Work out the finished part from the listing and answer in its coordinate system (mm). A direction names the side the tool comes from. Round coordinates to 2 decimals unless told otherwise and drop trailing zeros. Order: outer loops, then holes, each group sorted by start corner. A loop starts at its lowest first (then second) coordinate and runs counter-clockwise, first axis right, second up. Notation, with made-up numbers: (74.5, -26.75) -> (130.5, -26.75) arc R12 cw to (130.5, -20.75) -> close; hole circle Ø6 at (-38.75, 45.25). An arc over 180 degrees is marked (long way). Use one line per item in the form item = value.
```python
from build123d import *

# Parameters (mm, degrees)
F0_R     = 2
F2_W     = 4
F2_H     = 13
F3_DEPTH = 2
F5_DEPTH = 25


with BuildPart() as f1:
    # F0 (on Front) → F1 (revolve)
    with BuildSketch(Plane.XZ):
        with Locations((-18, 0)):
            Circle(F0_R)
    revolve(axis=Axis((0, 0, 11.250001), (0, 0, 1)))

    # F2 (on Top) → F3 (join, symmetric)
    with BuildSketch(Plane.XY):
        with Locations((2, -13.5)):
            Rectangle(F2_W, F2_H)
        with Locations((-2, -13.5)):
            Rectangle(F2_W, F2_H)
    extrude(amount=F3_DEPTH, both=True)

    # F4 (on face) → F5 (join)
    with BuildSketch(Plane.XZ.offset(20)):
        Polygon((0.5, 0.5), (2, 2), (0.5, 2), (0, 2), (-0.5, 2), (-2, 2), (-0.5, 0.5), (-0.5, -0.5), (-2, -2), (-0.5, -2), (0.5, -2), (2, -2), (0.5, -0.5), align=None)
        Polygon((2.070711, 1.929289), (2.141421, 2), (2, 2), (0.5, 0.5), (0.5, -0.5), (2, -2), (2.141421, -2), (2.070711, -1.929289), (0.6, -0.458579), (0.6, 0.458579), align=None)
        Polygon((-0.5, 0.5), (-2, 2), (-2.141421, 2), (-2.070711, 1.929289), (-0.6, 0.458579), (-0.6, -0.458579), (-2.070711, -1.929289), (-2.141421, -2), (-2, -2), (-0.5, -0.5), align=None)
    extrude(amount=F5_DEPTH)


solid = f1.part
```
Item 1: Consider line 1 along X through (y, z) = (-7.5, -1.1); line 2 along X through (y, z) = (-1, 1); line 3 along Y through (x, z) = (7, -0.6). Determine where each line is inside the solid, lowest interval first.
Findings:
line_1 = -18.18 to -14.51, -4 to 4, 14.51 to 18.18
line_2 = -19.71 to -16.24, 16.24 to 19.71
line_3 = -18.64 to -14.49, 14.49 to 18.64
Item 2: For faces 1 (the flat face through (0, -22, -2)), 2 (the flat face through (0, -7, 0)), 3 (the flat face through (-4, -19.8, 0.2)), 4 (the flat face through (0, -45, 0)), 5 (the flat face through (4, -19.8, 0.2)), determine the directions among +Z, -Z, +X, -X, +Y, -Y from which every point of the face is accessible in a straight line to the end or side of a thin tool.
Findings:
face_1 = -Z, +X, -X, +Y, -Y
face_2 = +Z, -Z
face_3 = -X, -Y
face_4 = +Z, -Z, +X, -X, -Y
face_5 = +X, -Y
Item 3: Flat-ended cylindrical pins translate along their axes: P1, Ø1.7, axis at x = -2, z = 0.5, coming from the -Y side; P2, Ø0.5, axis at y = -31.5, z = 0, coming from the -X side; P3, Ø1.2, axis at y = -10.5, z = 0, coming from the -X side. Find the tip coordinate at first contact, or state that the pin passes through.
Findings:
P1 = -20
P2 = -0.6
P3 = -17.38
Item 4: Determine the mould class of faces 6 (the flat face through (-4, -11, 0)), 7 (the flat face through (0, -22, 2)), 8 (the flat face through (3, -20, 0)) for opening direction Y: released by +Y, released by -Y, zero draft, split by the parting line, or undercut.
Findings:
face_6 = undercut
face_7 = zero draft
face_8 = released by -Y
Item 5: The part is cut by section A-A, the plane z = -1.25. Give the vertices of the cut face in (x, y), and give its area (3 significant figures).
Findings:
outline = (-4, -20) -> (-1.39, -20) -> (-1.39, -45) -> (1.39, -45) -> (1.39, -20) -> (4, -20) -> (4, -19.15) arc R19.56 ccw (long way) to (-4, -19.15) -> close; hole (-4, -15.94) -> (-4, -7) -> (4, -7) -> (4, -15.94) arc R16.44 ccw (long way) to start
area = 502 mm^2
Item 6: The part is cut by section B-B, the plane y = -8. Give the number of separate pieces and of enclosed holes in the cut face, and give its area (3 significant figures).
Findings:
separate_pieces = 3
enclosed_holes = 0
area = 60.1 mm^2
